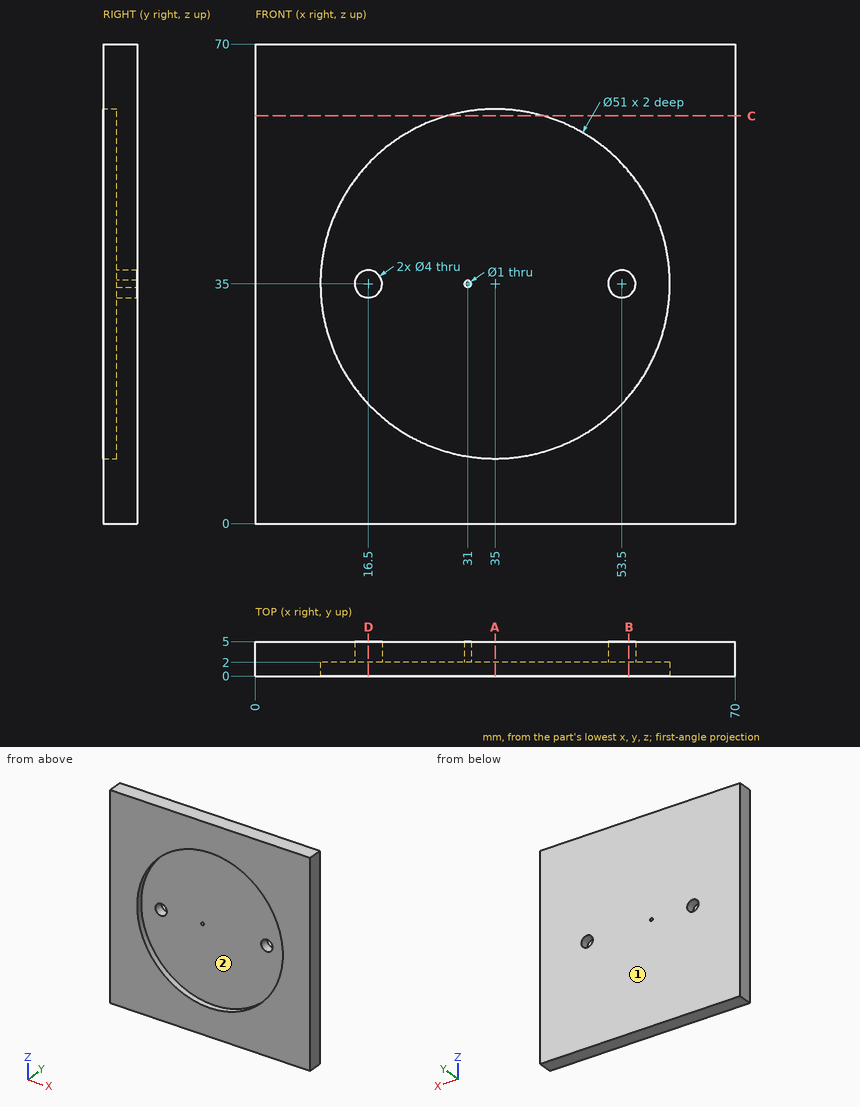
Input: dimensioned drawing with shaded views. Units: mm. Origin: part minimum x, y, z. Round coordinates to 2 decimals unless told otherwise and drop trailing zeros. Loops run counter-clockwise (first coordinate to the right, second up) from the corner with the lowest first, then second, coordinate; pieces in that order, holes last. Notation, with made-up numbers: M 26.25,-8.75 L 40.25,-8.75 A15 ccw 40.25,8.25 Z; hole C 14,59.5 d7. An arc over 180 degrees is marked long. Return JSON: item names as keys, results as strings. Group by question number.
1. Section query A-A on x = 35. Output: boundary loops of the cut face in (y, z).
2. Section query B-B on x = 54.5. Output: boundary loops of the cut face in (y, z).
3. Material intervals for line 1 along X through (y, z) = (4.2, 35); line 2 along Z through (x, y) = (31, 3.8); line 3 along X through (y, z) = (1.3, 35), sorted ascending. Write a range as from..to.
4. Section query C-C on z = 59.5. Output: boundary loops of the cut face in (x, y), and give its area (3 significant figures).
5. Section query D-D on x = 16.5. Output: boundary loops of the cut face in (y, z), and give its area (3 significant figures).
6. Mould query, pull axis X, two halves, no side actions, for the marked faces 1 and 2. Classes: released by +X, released by -X, zero draft, split by the parting line, or undercut.
7. Pin query (flat end, axial travel): pin 1 (3 mm diameter, centred on x = 53.5, z = 35, fed in from +Y). Return the tip coordinate at first contact, or that it passes through.
Checks:
{
 "1": {"outline": "M 0,0 L 5,0 L 5,70 L 0,70 L 0,60.5 L 2,60.5 L 2,9.5 L 0,9.5 Z"},
 "2": {"outline": "M 0,0 L 5,0 L 5,33.27 L 2,33.27 L 2,18.57 L 0,18.57 Z; M 0,51.43 L 2,51.43 L 2,36.73 L 5,36.73 L 5,70 L 0,70 Z"},
 "3": {"line 1": "x = 0..14.5, 18.5..30.5, 31.5..51.5, 55.5..70", "line 2": "z = 0..34.5, 35.5..70", "line 3": "x = 0..9.5, 60.5..70"},
 "4": {"outline": "M 0,0 L 27.93,0 L 27.93,2 L 42.07,2 L 42.07,0 L 70,0 L 70,5 L 0,5 Z", "area": "322 mm²"},
 "5": {"outline": "M 0,0 L 5,0 L 5,33 L 2,33 L 2,17.45 L 0,17.45 Z; M 0,52.55 L 2,52.55 L 2,37 L 5,37 L 5,70 L 0,70 Z", "area": "268 mm²"},
 "6": {"face 1": "zero draft", "face 2": "undercut"},
 "7": {"pin 1": "passes through"}
}
